Verification items for the finished model (mm, model axes). A direction names the side the tool comes from. Give positions to 0.01 mm unless a question says otherwise; leave off trailing zeros. Write each loop counter-clockwise with the first axis right and the second up, starting at its lowest first coordinate (ties: lowest second). Pieces come first, ordered by that corner, then holes. Notation, with made-up numbers: (-33, 10.25) - (20, 10.25) arc R18 ccw to (20, 24.25) - close; hole circle Ø3 at (27, 72.5). An arc over 180 degrees is marked (long way). Put each result on its own line as item: value.
from build123d import *

# Parameters (mm, degrees)
BOSS_EXTRUDE1_DEPTH = 41.2
SKETCH4_W           = 36.8
SKETCH4_H           = 61.2
CUT_EXTRUDE1_DEPTH  = 10000


with BuildPart() as part:
    # Sketch2 → Boss-Extrude1 (new body)
    with BuildSketch(Plane(origin=(0, 0, 0), x_dir=(0, 0, -1), z_dir=(1, 0, 0))):
        Polygon((0, 0), (-25, 0), (-25, 42.867109497), (-37.3, 61.2), (-37.3, 63.4), (0, 63.4), align=None)
    extrude(amount=BOSS_EXTRUDE1_DEPTH)

    # Sketch4 → Cut-Extrude1 (cut)
    with BuildSketch(Plane.XY):
        with Locations((20.6, 30.6)):
            Rectangle(SKETCH4_W, SKETCH4_H)
    extrude(amount=CUT_EXTRUDE1_DEPTH, mode=Mode.SUBTRACT)


solid = part.part
Q1. Set-up check for faces 4 (the face through (39, 30, 14)), 5 (the face through (1, 21, 25)), 6 (the face through (40, 0, 12)): record each of +Z, -Z, +X, -X, +Y, -Y from which the full face is reachable in a straight line by a thin tool's end or side.
Answers follow:
face 4: +Z, -Z, -Y
face 5: +Z, +X, -X, -Y
face 6: +Z, -Z, +X, -X, -Y
Q2. Section check B-B, the plane z = 14. Record the cut outline in (x, y).
Answers follow:
outline: (0, 0) - (2.2, 0) - (2.2, 61.2) - (39, 61.2) - (39, 0) - (41.2, 0) - (41.2, 63.4) - (0, 63.4) - close
Q3. Section check A-A, the plane y = 39. Record the cut outline in (x, z).
Answers follow:
outline: (0, 0) - (2.2, 0) - (2.2, 25) - (0, 25) - close; (39, 0) - (41.2, 0) - (41.2, 25) - (39, 25) - close
Q4. Section check D-D, the plane z = 30. Record the cut outline in (x, y).
Answers follow:
outline: (0, 50.32) - (2.2, 50.32) - (2.2, 61.2) - (39, 61.2) - (39, 50.32) - (41.2, 50.32) - (41.2, 63.4) - (0, 63.4) - close
Q5. Section check C-C, the plane x = 22. Record the cut outline in (y, z).
Answers follow:
outline: (61.2, 0) - (63.4, 0) - (63.4, 37.3) - (61.2, 37.3) - close
Q6. Go/stop test with flat-tipped pins: pin 1 Ø2.5 at (x, y) = (1.5, 20.5) entering from +Z; pin 2 Ø1 at (x, z) = (4.5, 9.5) entering from -Y. Record where each tip stops, or that it passes through.
Answers follow:
pin 1: stops at z = 25
pin 2: stops at y = 61.2
Q7. Release check for a two-part mould opening along X. For faces 1 (the face through (40, 21, 25)), 2 (the face through (41.2, 32, 14)), 3 (the face through (20, 61.2, 18)) record: released by +X, released by -X, zero draft, split by the parting line, or undercut.
Answers follow:
face 1: zero draft
face 2: released by +X
face 3: undercut
Q8. Scan lines: line 1 along X through (y, z) = (45.5, 8); line 2 along Y through (x, z) = (28.5, 13); line 3 along Y through (x, z) = (2, 29.5). Record each from-to range of solid material in increasing order.
Answers follow:
line 1: x = 0 to 2.2, 39 to 41.2
line 2: y = 61.2 to 63.4
line 3: y = 49.57 to 63.4
